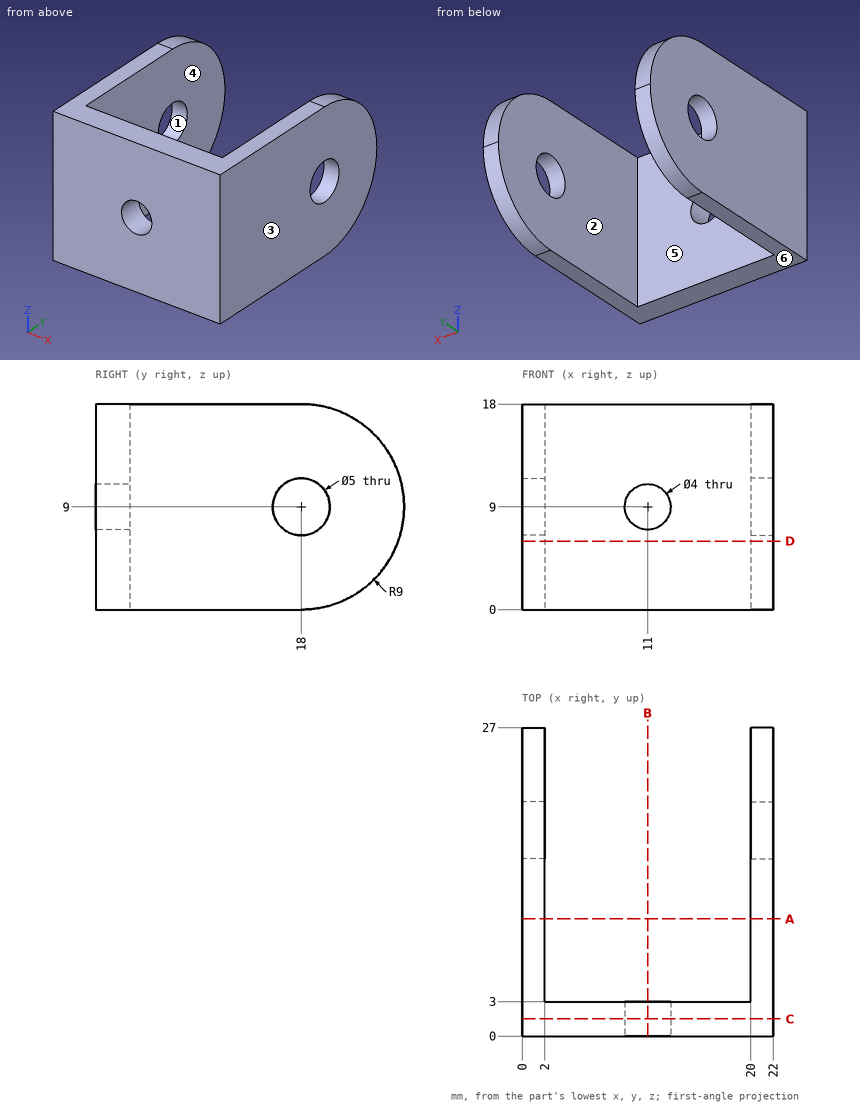
Geometry check sheet. Reference: drawing and pictorial views, mm from the part's lowest x, y, z. A direction names the side the tool comes from. Round coordinates to 2 decimals unless told otherwise and drop trailing zeros. Loops run counter-clockwise (first coordinate to the right, second up) from the corner with the lowest first, then second, coordinate; pieces in that order, holes last. Notation, with made-up numbers: (51, 8.25) - (79, 8.25) arc R12 ccw to (79, 18.25) - close; hole circle Ø3 at (24.5, -6). An arc over 180 degrees is marked (long way). Answer in a Markdown table with one row per item. Add a question column.
Q1. Tool access check on the marked faces 1 and 2. Record the directions out of +Z, -Z, +X, -X, +Y, -Y that give a thin tool (end or side, any length) a straight path to the whole face; none if there is none.
Q2. Material ranges on line 1 (X direction, y = 2.05, z = 9); line 2 (X direction, y = 10.5, z = 12.25); line 3 (Z direction, x = 21.35, y = 18), recorded low to high.
Q3. Section check C-C on y = 1.5. Enter the section's corners in (x, z), plus the area to 3 significant figures.
Q4. Section check A-A on y = 10.25. Enter the section's corners in (x, z).
Q5. Section check D-D on z = 6. Enter the section's corners in (x, y).
Q6. Gauge pin test, flat ends, axial feed: pin 1 (1.5 mm diameter, centred on x = 15.5, z = 15.5, fed in from -Y); pin 2 (6 mm diameter, centred on x = 2.5, z = 16, fed in from +Y); pin 3 (1 mm diameter, centred on x = 17, z = 15, fed in from +Y); pin 4 (3 mm diameter, centred on y = 18, z = 9, fed in from +X). Record the tip position at first contact, or that the pin passes through.
Q7. Section check B-B on x = 11. Enter the section's corners in (y, z), plus the area to 3 significant figures.
Q8. Release check for a two-part mould opening along X. For the marked faces 3, 4, 5 and 6 record: pulls with the +X half, pulls with the -X half, needs draft (parallel to the pull), parting line crosses it, or undercut.
Found:
| question | item | result |
|---|---|---|
| 1 | face 1 | +X, -X |
| 1 | face 2 | +Z, -Z, +Y |
| 2 | line 1 | x = 0 to 9, 13 to 22 |
| 2 | line 2 | x = 0 to 2, 20 to 22 |
| 2 | line 3 | z = 0 to 6.5, 11.5 to 18 |
| 3 | outline | (0, 0) - (22, 0) - (22, 18) - (0, 18) - close; hole circle Ø4 at (11, 9) |
| 3 | area | 383 mm² |
| 4 | outline | (0, 0) - (2, 0) - (2, 18) - (0, 18) - close; (20, 0) - (22, 0) - (22, 18) - (20, 18) - close |
| 5 | outline | (0, 0) - (22, 0) - (22, 26.49) - (20, 26.49) - (20, 3) - (2, 3) - (2, 26.49) - (0, 26.49) - close |
| 6 | pin 1 | stops at y = 0 |
| 6 | pin 2 | stops at y = 26.04 |
| 6 | pin 3 | stops at y = 3 |
| 6 | pin 4 | passes through |
| 7 | outline | (0, 0) - (3, 0) - (3, 7) - (0, 7) - close; (0, 11) - (3, 11) - (3, 18) - (0, 18) - close |
| 7 | area | 42.0 mm² |
| 8 | face 3 | pulls with the +X half |
| 8 | face 4 | undercut |
| 8 | face 5 | undercut |
| 8 | face 6 | needs draft |
